```python
from build123d import *

# Parameters (mm, degrees)
F1_DEPTH = 15.24
F3_DEPTH = 152.401
F5_DEPTH = 152.401


with BuildPart() as f1:
    # F0 (on Top) → F1 (new body)
    with BuildSketch(Plane.XY):
        Polygon((-68.542148, 76.080675), (-76.162148, 76.080675), (-76.162148, 68.460675), (-7.582148, -0.119325), (-76.162148, -68.699325), (-76.162148, -76.319325), (-68.542148, -76.319325), (0.037852, -7.739325), (68.617852, -76.319325), (76.237852, -76.319325), (76.237852, -68.699325), (7.657852, -0.119325), (76.237852, 68.460675), (76.237852, 76.080675), (68.617852, 76.080675), (0.037852, 7.500675), align=None)
    extrude(amount=F1_DEPTH)

    # F2 (on face) → F3 (cut, through all)
    with BuildSketch(Plane.XZ.offset(76.319325)):
        with BuildLine():
            Line((63.537852, 15.24), (-63.462148, 15.24))
            ThreePointArc((-63.462148, 15.24), (0.037852, 7.174442), (63.537852, 15.24))
        make_face()
    extrude(amount=-F3_DEPTH, mode=Mode.SUBTRACT)

    # F4 (on face) → F5 (cut, through all)
    with BuildSketch(Plane(origin=(-76.162148, 0, 0), x_dir=(0, -1, 0), z_dir=(-1, 0, 0))):
        with BuildLine():
            Line((63.619325, 15.24), (-63.380675, 15.24))
            ThreePointArc((-63.380675, 15.24), (0.119325, 7.174442), (63.619325, 15.24))
        make_face()
    extrude(amount=-F5_DEPTH, mode=Mode.SUBTRACT)


solid = f1.part
```
For this review, take the finished solid that the model builds, in its own axes (mm). A direction names the side the tool comes from. Coordinates: 2 decimals unless noted, no trailing zeros. Loops run counter-clockwise (first coordinate to the right, second up) from the corner with the lowest first, then second, coordinate; pieces in that order, holes last.
1. Mouldability with a two-part tool opening along Y and no side actions: class faces 1 (the flat face through (-42.35, -50.13, 5.82)), 2 (the flat face through (72, 76.081, 8)), 3 (the flat face through (50.05, -42.51, 5.82)) as +Y half, -Y half, draft (parallel to the pull), parting line (faces both ways), or undercut.
2. Add section D-D, the plane y = -41. Give the boundary of the cut face in (x, z), then the cut area to 3 significant figures.
3. Insertion check: P1, Ø1, axis at y = -53, z = 9.5, coming from the +X side; P2, Ø8, axis at y = -56, z = 7, coming from the -X side; P3, Ø4, axis at y = -5.5, z = 3.5, coming from the +X side. Each pin has a flat end and moves straight along its axis. Give the tip position at first contact, or say it passes through.
4. For line 1 (X direction, y = -42.5, z = 8.5); line 2 (Y direction, x = -28, z = 4.5); line 3 (Y direction, x = 12.5, z = 6.75), list the stretches that pass through material, from the lowest coordinate up.
5. For faces 4 (the flat face through (41.5, -49.2, 5.8)), 5 (the flat face through (76.238, 72, 8)), 6 (the flat face through (42.43, 49.89, 5.82)), 7 (the flat face through (-49.01, -41.55, 5.82)), list the 3-axis set-ups (+Z, -Z, +X, -X, +Y, -Y) from which the entire face can be reached by the end or side of a thin tool; tool diameter is ignored.
6. Add section A-A, the plane x = 38. Give the boundary of the cut face in (y, z).
7. Add section C-C, the plane z = 2. Give the boundary of the cut face in (x, y), then the cut area to 3 significant figures.
Result:
1. face 1: -Y half
1. face 2: +Y half
1. face 3: undercut
2. outline: (-48.46, 0) - (-33.22, 0) - (-33.22, 9.36) arc R254 cw to (-40.84, 10.49) - (-48.46, 10.49) - close; (33.3, 0) - (48.54, 0) - (48.54, 10.49) - (40.92, 10.49) arc R254 cw to (33.3, 9.36) - close
2. area: 311 mm2
3. P1: stops at x = 61.04
3. P2: stops at x = -67.46
3. P3: stops at x = 15.04
4. line 1: x = -49.96 to -34.72, 34.8 to 50.04
4. line 2: y = -35.78 to -20.54, 20.3 to 35.54
4. line 3: y = -20.2 to -4.96, 4.72 to 19.96
5. face 4: +Z, -Z, -Y
5. face 5: +Z, -Z, +X, +Y, -Y
5. face 6: +Z, -Z, +Y
5. face 7: +Z, -Z, -X
6. outline: (-45.7, 0) - (-30.46, 0) - (-30.46, 8.99) arc R254 cw to (-38.08, 10.03) - (-45.7, 10.03) - close; (30.22, 0) - (45.46, 0) - (45.46, 10.03) - (37.84, 10.03) arc R254 cw to (30.22, 8.99) - close
7. outline: (-76.16, -76.32) - (-68.54, -76.32) - (0.04, -7.74) - (68.62, -76.32) - (76.24, -76.32) - (76.24, -68.7) - (7.66, -0.12) - (76.24, 68.46) - (76.24, 76.08) - (68.62, 76.08) - (0.04, 7.5) - (-68.54, 76.08) - (-76.16, 76.08) - (-76.16, 68.46) - (-7.58, -0.12) - (-76.16, -68.7) - close
7. area: 4,410 mm2
